```python
from build123d import *

# Parameters (mm, degrees)
SKETCH1_W           = 12.7
SKETCH1_H           = 12.7
BOSS_EXTRUDE1_DEPTH = 9.525
SKETCH3_W           = 3.048
SKETCH3_H           = 3.048
BOSS_EXTRUDE2_DEPTH = 9.525
SKETCH4_R           = 3.175
CUT_EXTRUDE1_DEPTH  = 6.35


with BuildPart() as part:
    # Sketch1 → Boss-Extrude1 (new body)
    with BuildSketch(Plane(origin=(0, 0, 0), x_dir=(1, 0, 0), z_dir=(0, 1, 0))):
        Rectangle(SKETCH1_W, SKETCH1_H)
    extrude(amount=BOSS_EXTRUDE1_DEPTH)

    # Sketch3 → Boss-Extrude2 (add)
    with BuildSketch(Plane(origin=(0, 9.525, 0), x_dir=(1, 0, 0), z_dir=(0, 1, 0))):
        Rectangle(SKETCH3_W, SKETCH3_H)
    extrude(amount=BOSS_EXTRUDE2_DEPTH)

    # Sketch4 → Cut-Extrude1 (cut)
    with BuildSketch(Plane.XZ):
        with Locations(Location((0, 0, 0), (0, 0, 270))):
            Circle(SKETCH4_R)
    extrude(amount=-CUT_EXTRUDE1_DEPTH, mode=Mode.SUBTRACT)


solid = part.part
```
Design review of the part built by this model. Coordinates are the model's own, in mm. A direction names the side the tool comes from. Coordinates: 2 decimals unless noted, no trailing zeros. Loops run counter-clockwise (first coordinate to the right, second up) from the corner with the lowest first, then second, coordinate; pieces in that order, holes last. Notation, with made-up numbers: (18.25, 72.5) - (72.25, 72.5) arc R26 cw to (72.25, 99.5) - close; hole circle Ø10 at (-28.5, 72). An arc over 180 degrees is marked (long way). Use CSV: the item, a comma, the result in double quotes. Start each with the question number.
1) Consider section C-C on y = 12.5. Write out the cut boundary in (x, z).
2) The part is to be moulded in two halves that separate along X. For faces 4 (the flat face through (0, 14, 1.524)), 5 (the cylindrical face through (-1.93, 3.13, 2.52)), 6 (the flat face through (-1.524, 14, 0)), 7 (the flat face through (1.524, 14, 0)), say which applies: +X half, -X half, draft (parallel to the pull), parting line (faces both ways), or undercut.
3) Consider section A-A on z = 0. Write out the cut boundary in (x, y) (3 decimals), then the cut area to 3 significant figures.
4) For pin 1 Ø1 at (x, z) = (-1.5, 2.5) entering from +Y (3 decimals); pin 2 Ø0.9 at (x, y) = (0.5, 14) entering from +Z; pin 3 Ø2.5 at (x, y) = (0.5, 13.5) entering from -Z; pin 4 Ø6 at (y, z) = (16, -5) entering from +X, all flat-tipped, find the tip position at first contact; note any pin that passes through.
5) Consider section B-B on x = -2.5. Write out the cut boundary in (y, z) (3 decimals), then the cut area to 3 significant figures.
6) Consider section D-D on x = 0. Write out the cut boundary in (y, z) (3 decimals), then the cut area to 3 significant figures.
7) Tool access review of faces 1 (the flat face through (-6.35, 5, 0)), 2 (the flat face through (0, 14, -1.524)), 3 (the flat face through (0, 6.35, 0)): name each direction out of +Z, -Z, +X, -X, +Y, -Y from which nothing blocks a thin tool from reaching the whole face with its end or side.
8) Wall thickness on L1, parallel to X at y = 4.25, z = 0 (3 decimals); L2, parallel to Y at x = 4.5, z = 0 (3 decimals); L3, parallel to X at y = 5.5, z = 1.75: over which ranges is each line inside the solid? List them lowest first. Write a range as from..to.
Geometry says:
1,outline,"(-1.52, -1.52) - (1.52, -1.52) - (1.52, 1.52) - (-1.52, 1.52) - close"
2,face 4,"draft"
2,face 5,"undercut"
2,face 6,"-X half"
2,face 7,"+X half"
3,outline,"(-6.35, 0) - (-3.175, 0) - (-3.175, 6.35) - (3.175, 6.35) - (3.175, 0) - (6.35, 0) - (6.35, 9.525) - (1.524, 9.525) - (1.524, 19.05) - (-1.524, 19.05) - (-1.524, 9.525) - (-6.35, 9.525) - close"
3,area,"110 mm^2"
4,pin 1,"y = 9.525"
4,pin 2,"z = 1.52"
4,pin 3,"z = -1.52"
4,pin 4,"through"
5,outline,"(0, -6.35) - (9.525, -6.35) - (9.525, 6.35) - (0, 6.35) - (0, 1.957) - (6.35, 1.957) - (6.35, -1.957) - (0, -1.957) - close"
5,area,"96.1 mm^2"
6,outline,"(0, -6.35) - (9.525, -6.35) - (9.525, -1.524) - (19.05, -1.524) - (19.05, 1.524) - (9.525, 1.524) - (9.525, 6.35) - (0, 6.35) - (0, 3.175) - (6.35, 3.175) - (6.35, -3.175) - (0, -3.175) - close"
6,area,"110 mm^2"
7,face 1,"+Z, -Z, -X, +Y, -Y"
7,face 2,"-Z, +X, -X, +Y"
7,face 3,"-Y"
8,L1,"-6.35..-3.175, 3.175..6.35"
8,L2,"0..9.525"
8,L3,"-6.35..-2.65, 2.65..6.35"
